Geometry check sheet. Reference: drawing and pictorial views, mm from the part's lowest x, y, z. A direction names the side the tool comes from. Give positions to 0.01 mm unless a question says otherwise; leave off trailing zeros. Loops run counter-clockwise (first coordinate to the right, second up) from the corner with the lowest first, then second, coordinate; pieces in that order, holes last. Notation, with made-up numbers: (-1.75, 59) - (43.25, 59) arc R22 cw to (43.25, 75) - close; hole circle Ø2 at (19.5, 45.25). An arc over 180 degrees is marked (long way). One line per question, with ' | ' between items. Start each with the question number.
1. Section check B-B, the plane x = 24.5. Enter the section's corners in (y, z), then the cut area to 3 significant figures.
2. Section check C-C, the plane y = 72.05. Enter the section's corners in (x, z) (1 decimal).
3. Section check A-A, the plane y = 36.5. Enter the section's corners in (x, z), then the cut area to 3 significant figures.
4. Mould release check, pull along Y, two halves, no side actions. Record for the marked faces 1, 2, 3 and 4: +Y half, -Y half, draft (parallel to the pull), parting line (faces both ways), or undercut.
5. Thickness scan on line 1 along Z through (x, y) = (0.6, 72.05) (1 decimal); line 2 along X through (y, z) = (52, 24.5); line 3 along Y through (x, z) = (34, 36). Record the ranges inside material, lowest first. Write a range as from..to.
6. Depth check by flat-ended pin: pin 1 Ø1 at (x, z) = (18.5, 0.5) entering from -Y; pin 2 Ø19.5 at (x, z) = (19, 11) entering from +Y; pin 3 Ø5 at (y, z) = (72.05, 28.42) entering from -X; pin 4 Ø4 at (y, z) = (3, 28) entering from +X. Enter the tip coordinate at first touch or a pass-through.
7. Tool access check on the marked faces 5, 6 and 7. Record the directions out of +Z, -Z, +X, -X, +Y, -Y that give a thin tool (end or side, any length) a straight path to the whole face; none if there is none.
8. Section check D-D, the plane z = 32. Enter the section's corners in (x, y).
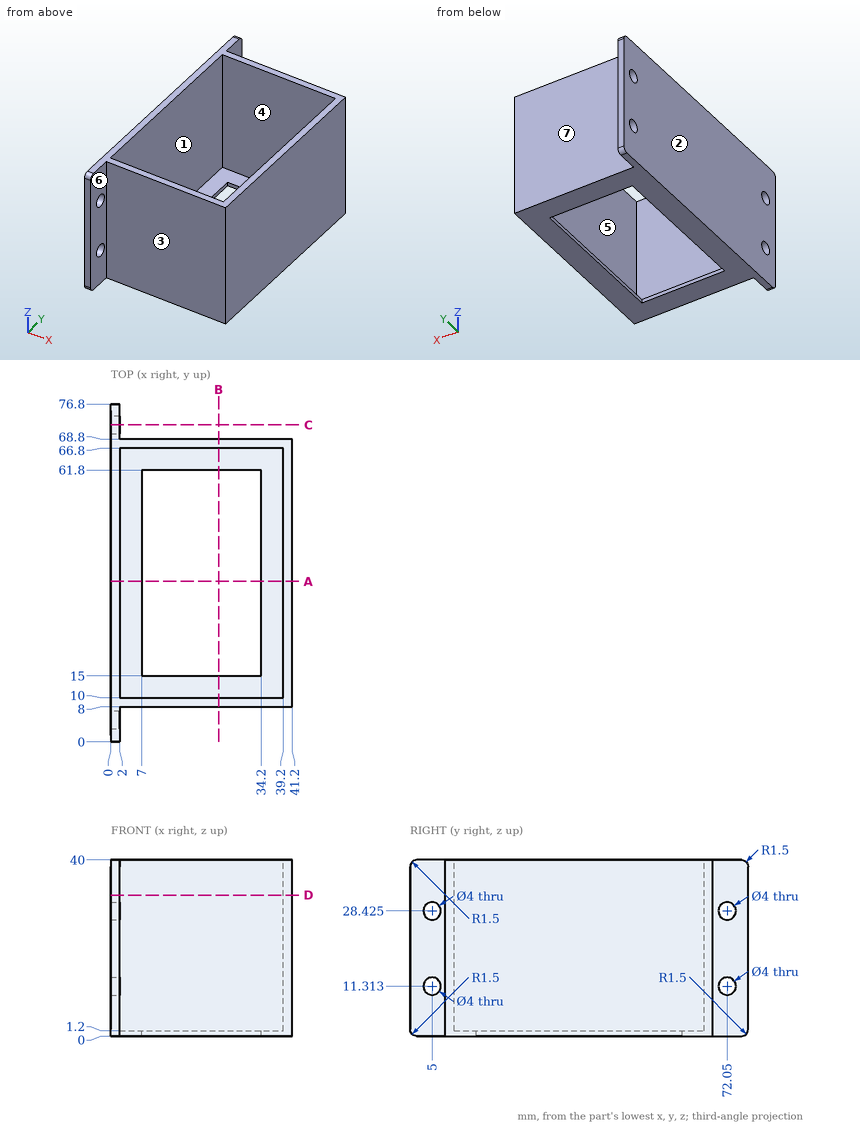
Results list:
1) outline: (8, 0) - (15, 0) - (15, 1.2) - (10, 1.2) - (10, 40) - (8, 40) - close; (61.8, 0) - (68.8, 0) - (68.8, 40) - (66.8, 40) - (66.8, 1.2) - (61.8, 1.2) - close | area: 172 mm²
2) outline: (0, 0) - (2, 0) - (2, 9.3) - (0, 9.3) - close; (0, 13.3) - (2, 13.3) - (2, 26.4) - (0, 26.4) - close; (0, 30.4) - (2, 30.4) - (2, 40) - (0, 40) - close
3) outline: (0, 0) - (7, 0) - (7, 1.2) - (2, 1.2) - (2, 40) - (0, 40) - close; (34.2, 0) - (41.2, 0) - (41.2, 40) - (39.2, 40) - (39.2, 1.2) - (34.2, 1.2) - close | area: 172 mm²
4) face 1: undercut | face 2: draft | face 3: -Y half | face 4: undercut
5) line 1: 0..9.3, 13.3..26.4, 30.4..40 | line 2: 0..2, 39.2..41.2 | line 3: 8..10, 66.8..68.8
6) pin 1: y = 8 | pin 2: y = 68.8 | pin 3: x = 0 | pin 4: x = 2
7) face 5: +Z | face 6: +Z, -Z, +X, -Y | face 7: +Z, -Z, +X, +Y
8) outline: (0, 0) - (2, 0) - (2, 8) - (41.2, 8) - (41.2, 68.8) - (2, 68.8) - (2, 76.8) - (0, 76.8) - close; hole (2, 10) - (39.2, 10) - (39.2, 66.8) - (2, 66.8) - close
